from build123d import *


with BuildPart() as f1:
    # F0 (on Front) → F1 (revolve)
    with BuildSketch(Plane.XZ):
        with BuildLine():
            Line((26.958548, 0), (0, 0))
            Line((0, 0), (0, -2))
            Line((0, -2), (28.113249, -2))
            ThreePointArc((28.113249, -2), (30.613249, -1.330127), (32.443376, 0.5))
            Line((32.443376, 0.5), (48.064948, 27.557357))
            ThreePointArc((48.064948, 27.557357), (48.180461, 28.248623), (47.81385, 28.84594))
            ThreePointArc((47.81385, 28.84594), (47.007656, 29.038895), (46.332897, 28.557357))
            Line((46.332897, 28.557357), (31.288675, 2.5))
            ThreePointArc((31.288675, 2.5), (29.458548, 0.669873), (26.958548, 0))
        make_face()
    revolve(axis=Axis((0, 0, 22.936326), (0, 0, 1)))


solid = f1.part
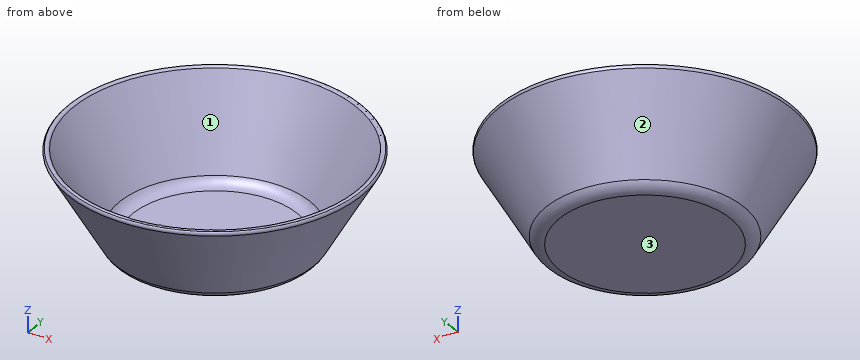
Model file for the job. Use its own axes, mm. Face numbers are marked on the shaded views. Give positions to 0.01 mm unless a question says otherwise; leave off trailing zeros. Loops run counter-clockwise (first coordinate to the right, second up) from the corner with the lowest first, then second, coordinate; pieces in that order, holes last.
1) Pull direction Y, two halves, no side cores. Call the marked faces 1, 2 and 3: +Y half, -Y half, draft (parallel to the pull), parting line (faces both ways), or undercut.
2) Saw through at A-A (x = 0). Write the cut outline in (y, z).
3) Saw through at D-D (z = 24.5). Write the cut outline in (x, y).
4) Wall check: line 1 (Z direction, x = 6, y = 4); line 2 (X direction, y = 18, z = 26); line 3 (X direction, y = 19, z = 21). Give the ranges that are in metal, low to high.
5) Flat gauge pins, fed straight in: pin 1 Ø16 at (x, y) = (0.5, 4.5) entering from +Z; pin 2 Ø4 at (y, z) = (-19.5, 23.5) entering from -X; pin 3 Ø1 at (y, z) = (1, 4) entering from -X. Where does each tip first touch, or does it go through?
6) Saw through at C-C (z = 12). Write the cut outline in (x, y).
Answer block:
1. face 1: undercut
1. face 2: parting line
1. face 3: draft
2. outline: (-48.06, 27.56) - (-32.44, 0.5) arc R5 ccw to (-28.11, -2) - (28.11, -2) arc R5 ccw to (32.44, 0.5) - (48.06, 27.56) arc R1 ccw to (47.81, 28.85) arc R1 ccw to (46.33, 28.56) - (31.29, 2.5) arc R5 cw to (26.96, 0) - (-26.96, 0) arc R5 cw to (-31.29, 2.5) - (-46.33, 28.56) arc R1 ccw to (-47.81, 28.85) arc R1 ccw to start
3. outline: circle Ø92.6 at (0, 0); hole circle Ø87.98 at (0, 0)
4. line 1: z = -2 to 0
4. line 2: x = -43.6 to -41.09, 41.09 to 43.6
4. line 3: x = -40 to -37.42, 37.42 to 40
5. pin 1: stops at z = 0
5. pin 2: stops at x = -42.91
5. pin 3: stops at x = -34.74
6. outline: circle Ø78.17 at (0, 0); hole circle Ø73.55 at (0, 0)
